```python
from build123d import *

# Parameters (mm, degrees)
SKETCH1_R           = 27
BOSS_EXTRUDE1_DEPTH = 5
SKETCH3_R           = 17.45
BOSS_EXTRUDE2_DEPTH = 6.5
SKETCH4_R           = 11
CUT_EXTRUDE1_DEPTH  = 7
SKETCH7_R           = 1.5
CUT_EXTRUDE2_DEPTH  = 40.877938763
SKETCH8_R           = 7.5
CUT_EXTRUDE3_DEPTH  = 40.877938763
CHAMFER1_SIZE       = 1.3
SKETCH9_R           = 2.4
CUT_EXTRUDE4_DEPTH  = 15
CUT_EXTRUDE5_REACH  = 41.878
SKETCH10_R          = 2


with BuildPart() as part:
    # Sketch1 → Boss-Extrude1 (new body)
    with BuildSketch(Plane(origin=(0, 0, 0), x_dir=(1, 0, 0), z_dir=(0, 1, 0))):
        with Locations(Location((0, 0, 0), (0, 0, 270))):
            Circle(SKETCH1_R)
    extrude(amount=BOSS_EXTRUDE1_DEPTH)

    # Sketch3 → Boss-Extrude2 (add)
    with BuildSketch(Plane(origin=(0, 5, 0), x_dir=(1, 0, 0), z_dir=(0, 1, 0))):
        with Locations(Location((0, 0, 0), (0, 0, 90))):
            Circle(SKETCH3_R)
    extrude(amount=BOSS_EXTRUDE2_DEPTH)

    # Sketch4 → Cut-Extrude1 (cut)
    with BuildSketch(Plane.XZ):
        with Locations(Location((0, 0, 0), (0, 0, 270))):
            Circle(SKETCH4_R)
    extrude(amount=-CUT_EXTRUDE1_DEPTH, mode=Mode.SUBTRACT)

    # Sketch7 → Cut-Extrude2 (cut, through all)
    with BuildSketch(Plane.XZ):
        with Locations(Location((-15.5, 15.5, 0), (0, 0, 270))):
            Circle(SKETCH7_R)
        with Locations(Location((15.5, 15.5, 0), (0, 0, 270))):
            Circle(SKETCH7_R)
        with Locations(Location((15.5, -15.5, 0), (0, 0, 270))):
            Circle(SKETCH7_R)
        with Locations(Location((-15.5, -15.5, 0), (0, 0, 270))):
            Circle(SKETCH7_R)
    extrude(amount=-CUT_EXTRUDE2_DEPTH, mode=Mode.SUBTRACT)

    # Sketch8 → Cut-Extrude3 (cut, through all)
    with BuildSketch(Plane(origin=(0, 11.5, 0), x_dir=(1, 0, 0), z_dir=(0, 1, 0))):
        with Locations(Location((0, 0, 0), (0, 0, 270))):
            Circle(SKETCH8_R)
    extrude(amount=-CUT_EXTRUDE3_DEPTH, mode=Mode.SUBTRACT)

    # Chamfer1
    chamfer1_edges = [part.edges().sort_by_distance(p)[0] for p in [
        (-15.5, 5, -14),
        (15.5, 5, -14),
        (15.5, 5, 17),
        (-15.5, 5, 17),
    ]]
    chamfer(chamfer1_edges, length=CHAMFER1_SIZE)

    # Sketch9 → Cut-Extrude4 (cut)
    with BuildSketch(Plane(origin=(0, 11.5, 0), x_dir=(1, 0, 0), z_dir=(0, 1, 0))):
        with Locations(Location((0, 15, 0), (0, 0, 270))):
            Circle(SKETCH9_R)
        with Locations(Location((12.990381057, 7.5, 0), (0, 0, 270))):
            Circle(SKETCH9_R)
        with Locations(Location((12.990381057, -7.5, 0), (0, 0, 270))):
            Circle(SKETCH9_R)
        with Locations(Location((0, -15, 0), (0, 0, 270))):
            Circle(SKETCH9_R)
        with Locations(Location((-12.990381057, -7.5, 0), (0, 0, 270))):
            Circle(SKETCH9_R)
        with Locations(Location((-12.990381057, 7.5, 0), (0, 0, 270))):
            Circle(SKETCH9_R)
    extrude(amount=-CUT_EXTRUDE4_DEPTH, mode=Mode.SUBTRACT)

    # Sketch10 → Cut-Extrude5 (cut, up to next)
    with BuildSketch(Plane.XZ, mode=Mode.PRIVATE) as cut_extrude5_sk1:
        with Locations(Location((4.633375967, 9.976563895, 0), (0, 0, 329.872709141))):
            Circle(SKETCH10_R)
    cut_extrude5_tool1 = extrude(cut_extrude5_sk1.sketch, amount=-CUT_EXTRUDE5_REACH, mode=Mode.PRIVATE) & part.part
    # Sketch10 → Cut-Extrude5 (cut, up to next)
    with BuildSketch(Plane.XZ, mode=Mode.PRIVATE) as cut_extrude5_sk2:
        with Locations(Location((10.956645759, 0.975660655, 0), (0, 0, 269.872709141))):
            Circle(SKETCH10_R)
    cut_extrude5_tool2 = extrude(cut_extrude5_sk2.sketch, amount=-CUT_EXTRUDE5_REACH, mode=Mode.PRIVATE) & part.part
    # Sketch10 → Cut-Extrude5 (cut, up to next)
    with BuildSketch(Plane.XZ, mode=Mode.PRIVATE) as cut_extrude5_sk3:
        with Locations(Location((6.323269792, -9.00090324, 0), (0, 0, 209.872709141))):
            Circle(SKETCH10_R)
    cut_extrude5_tool3 = extrude(cut_extrude5_sk3.sketch, amount=-CUT_EXTRUDE5_REACH, mode=Mode.PRIVATE) & part.part
    # Sketch10 → Cut-Extrude5 (cut, up to next)
    with BuildSketch(Plane.XZ, mode=Mode.PRIVATE) as cut_extrude5_sk4:
        with Locations(Location((-4.633375967, -9.976563895, 0), (0, 0, 340.304526282))):
            Circle(SKETCH10_R)
    cut_extrude5_tool4 = extrude(cut_extrude5_sk4.sketch, amount=-CUT_EXTRUDE5_REACH, mode=Mode.PRIVATE) & part.part
    # Sketch10 → Cut-Extrude5 (cut, up to next)
    with BuildSketch(Plane.XZ, mode=Mode.PRIVATE) as cut_extrude5_sk5:
        with Locations(Location((-10.956645759, -0.975660655, 0), (0, 0, 280.304526282))):
            Circle(SKETCH10_R)
    cut_extrude5_tool5 = extrude(cut_extrude5_sk5.sketch, amount=-CUT_EXTRUDE5_REACH, mode=Mode.PRIVATE) & part.part
    # Sketch10 → Cut-Extrude5 (cut, up to next)
    with BuildSketch(Plane.XZ, mode=Mode.PRIVATE) as cut_extrude5_sk6:
        with Locations(Location((-6.323269792, 9.00090324, 0), (0, 0, 220.304526282))):
            Circle(SKETCH10_R)
    cut_extrude5_tool6 = extrude(cut_extrude5_sk6.sketch, amount=-CUT_EXTRUDE5_REACH, mode=Mode.PRIVATE) & part.part
    add(cut_extrude5_tool1.solids().sort_by_distance((4.633376, 0, 9.976564))[0], mode=Mode.SUBTRACT)
    add(cut_extrude5_tool2.solids().sort_by_distance((10.956646, 0, 0.975661))[0], mode=Mode.SUBTRACT)
    add(cut_extrude5_tool3.solids().sort_by_distance((6.32327, 0, -9.000903))[0], mode=Mode.SUBTRACT)
    add(cut_extrude5_tool4.solids().sort_by_distance((-4.633376, 0, -9.976564))[0], mode=Mode.SUBTRACT)
    add(cut_extrude5_tool5.solids().sort_by_distance((-10.956646, 0, -0.975661))[0], mode=Mode.SUBTRACT)
    add(cut_extrude5_tool6.solids().sort_by_distance((-6.32327, 0, 9.000903))[0], mode=Mode.SUBTRACT)


solid = part.part
```
Can you work these out from the model? Positions are in its coordinate system, mm. A direction names the side the tool comes from. Round coordinates to 2 decimals unless told otherwise and drop trailing zeros. Loops run counter-clockwise (first coordinate to the right, second up) from the corner with the lowest first, then second, coordinate; pieces in that order, holes last. Notation, with made-up numbers: M 10.5,42 L 32.5,42 A22 cw 32.5,53 Z; hole C 77,-29 d9. An arc over 180 degrees is marked long. Write item = value, one per line. Start each with the question number.
(1) Suppose I cut it at D-D on z = -21. Write out the boundary of the cut face in (x, y).
(2) I'm going to push flat-ended pins straight in: P1, Ø5, axis at x = 8, y = 1, coming from the -Z side; P2, Ø1, axis at x = 20, y = 2.5, coming from the -Z side; P3, Ø11, axis at x = 3, z = -0.5, coming from the -Y side. Where does each tip first touch, or does it pass through?
(3) If we mould it in two halves opening along Z, with no side actions, what happens to faces 3 (the face through (15.481, 8.204, -8.052)), 4 (the face through (0, 5, 18)), 5 (the face through (7.54, 6.95, -10.59))? For each: released by +Z, released by -Z, zero draft, split by the parting line, or undercut.
(4) Suppose I cut it at A-A on x = 0. Write out the boundary of the cut face in (y, z), plus the area to 3 significant figures.
(5) I need wall thicknesses on line 1 along Z through (x, y) = (-3, 10.75); line 2 along X through (y, z) = (1.5, -15.5); line 3 along X through (y, z) = (6.5, 6.5). Which ranges of each line are inside material? Lowest first, please.
(6) Suppose I cut it at B-B on z = 15.5. Write out the boundary of the cut face in (x, y).
(7) Which directions (+Z, -Z, +X, -X, +Y, -Y) give clear straight access to the entire face, cutting with the end or side of a thin tool? Please do faces 1 (the face through (-26.36, 2.46, -5.85)), 2 (the face through (0.92, 3.45, -10.96)).
(8) Suppose I cut it at C-C on y = 6.25. Write out the boundary of the cut face in (x, z).
Answer block:
q1.outline = M -16.97,0 L 16.97,0 L 16.97,5 L -16.97,5 Z
q2.P1 = -26.43
q2.P2 = -18.67
q2.P3 = 7
q3.face_3 = split by the parting line
q3.face_4 = zero draft
q3.face_5 = undercut
q4.outline = M 0,-27 L 5,-27 L 5,-17.45 L 11.5,-17.45 L 11.5,-17.4 L 0,-17.4 Z; M 0,-12.6 L 11.5,-12.6 L 11.5,-7.5 L 7,-7.5 L 7,-11 L 0,-11 Z; M 0,11 L 7,11 L 7,7.5 L 11.5,7.5 L 11.5,12.6 L 0,12.6 Z; M 0,17.4 L 11.5,17.4 L 11.5,17.45 L 5,17.45 L 5,27 L 0,27 Z
q4.area = 165 mm²
q5.line_1 = -17.19 to -11.13, -8.82 to -6.87, 6.87 to 17.19
q5.line_2 = -22.11 to -17, -14 to -2.35, 2.35 to 14, 17 to 22.11
q5.line_3 = -16.19 to -15.17, -10.81 to -8.87, 8.87 to 10.81, 15.17 to 16.19
q6.outline = M -22.11,0 L -17,0 L -17,3.7 L -18.3,5 L -22.11,5 Z; M -14,0 L -2.35,0 L -2.35,11.5 L -8.02,11.5 L -8.02,5 L -12.7,5 L -14,3.7 Z; M 2.35,0 L 14,0 L 14,3.7 L 12.7,5 L 8.02,5 L 8.02,11.5 L 2.35,11.5 Z; M 17,0 L 22.11,0 L 22.11,5 L 18.3,5 L 17,3.7 Z
q7.face_1 = +Y, -Y
q7.face_2 = -Y
q8.outline = C 0,0 d34.9; hole C -12.99,-7.5 d4.8; hole C -12.99,7.5 d4.8; hole M -10.95,1.02 A2 ccw long -10.6,-2.94 A11 ccw -6.36,-8.97 A2 ccw long -2.75,-10.65 A11 ccw 4.59,-10 A2 ccw long 7.85,-7.71 A11 ccw 10.95,-1.02 A2 ccw long 10.6,2.94 A11 ccw 6.36,8.97 A2 ccw long 2.75,10.65 A11 ccw -4.59,10 A2 ccw long -7.85,7.71 A11 ccw Z; hole C 0,-15 d4.8; hole C 0,15 d4.8; hole C 12.99,-7.5 d4.8; hole C 12.99,7.5 d4.8
